from build123d import *

# Parameters (mm, degrees)
CUT_EXTRUDE2_DEPTH      = 10
CUT_EXTRUDE2_DEPTH_BACK = 10
BOSS_EXTRUDE1_START     = -0.2
SKETCH6_R               = 2.5
SKETCH6_R_2             = 1.5
BOSS_EXTRUDE1_DEPTH     = 10


with BuildPart() as part:
    # Sketch1 → Revolve1 (revolve)
    with BuildSketch(Plane(origin=(0, 0, 0), x_dir=(0, 0, -1), z_dir=(1, 0, 0)), mode=Mode.PRIVATE) as revolve1_sk:
        Polygon((6.5, 15.5), (-6.5, 15.5), (-8, 17), (-8, 18.5), (-6.5, 18.5), (-5, 16.5), (5, 16.5), (6.5, 18.5), (8, 18.5), (8, 17), align=None)
    revolve(revolve1_sk.sketch.rotate(Axis((0, 0, 10.557897078), (0, 0, -1)), 90), axis=Axis((0, 0, 10.557897078), (0, 0, -1)))

    # Sketch3 → Revolve2 (revolve)
    with BuildSketch(Plane(origin=(0, 0, 0), x_dir=(0, 0, -1), z_dir=(1, 0, 0)), mode=Mode.PRIVATE) as revolve2_sk:
        with BuildLine():
            Line((-6.25, 4.5), (-6.25, 2.5))
            Line((-6.25, 2.5), (-4.75, 2.5))
            Line((-4.75, 2.5), (-4.75, 0))
            Line((-4.75, 0), (-4, 0))
            Line((-4, 0), (-4, 2.5))
            Line((-4, 2.5), (5.75, 2.5))
            Line((5.75, 2.5), (5.75, 3.25))
            Line((5.75, 3.25), (-5.5, 3.25))
            Line((-5.5, 3.25), (-5.5, 4.5))
            ThreePointArc((-5.5, 4.5), (-7.225700509, 9.988531242), (-6.719669914, 15.719669914))
            Line((-6.719669914, 15.719669914), (-7.25, 16.25))
            ThreePointArc((-7.25, 16.25), (-7.918610158, 10.275543816), (-6.25, 4.5))
        make_face()
    revolve(revolve2_sk.sketch.rotate(Axis((0, 0, 4.75), (0, 0, -1)), 90), axis=Axis((0, 0, 4.75), (0, 0, -1)))

    # Sketch4 → Cut-Extrude2 (cut, two sides: drawn at the far end of the back side and taken through both)
    with BuildSketch(Plane.XY.offset(-CUT_EXTRUDE2_DEPTH_BACK)):
        with BuildLine():
            Line((-1.5, 7.406883651), (-8.150991135, 14.057874786))
            ThreePointArc((-8.150991135, 14.057874786), (0, 16.25), (8.150991135, 14.057874786))
            Line((8.150991135, 14.057874786), (1.5, 7.406883651))
            ThreePointArc((1.5, 7.406883651), (0, 7.557243242), (-1.5, 7.406883651))
        make_face()
        with BuildLine():
            Line((6.58083947, 3.715437698), (10.851038639, 12.096175447))
            ThreePointArc((10.851038639, 12.096175447), (15.45466839, 5.021526159), (15.888628203, -3.40793102))
            Line((15.888628203, -3.40793102), (7.507890453, 0.862268149))
            ThreePointArc((7.507890453, 0.862268149), (7.187365431, 2.335316592), (6.58083947, 3.715437698))
        make_face()
        with BuildLine():
            Line((5.567182467, -5.110616871), (14.857301828, -6.582027226))
            ThreePointArc((14.857301828, -6.582027226), (9.55151035, -13.146526159), (1.668721129, -16.164091988))
            Line((1.668721129, -16.164091988), (3.140131484, -6.873972628))
            ThreePointArc((3.140131484, -6.873972628), (4.442036126, -6.113938214), (5.567182467, -5.110616871))
        make_face()
        with BuildLine():
            Line((-3.140131484, -6.873972628), (-1.668721129, -16.164091988))
            ThreePointArc((-1.668721129, -16.164091988), (-9.55151035, -13.146526159), (-14.857301828, -6.582027226))
            Line((-14.857301828, -6.582027226), (-5.567182467, -5.110616871))
            ThreePointArc((-5.567182467, -5.110616871), (-4.442036126, -6.113938214), (-3.140131484, -6.873972628))
        make_face()
        with BuildLine():
            Line((-7.507890453, 0.862268149), (-15.888628203, -3.40793102))
            ThreePointArc((-15.888628203, -3.40793102), (-15.45466839, 5.021526159), (-10.851038639, 12.096175447))
            Line((-10.851038639, 12.096175447), (-6.58083947, 3.715437698))
            ThreePointArc((-6.58083947, 3.715437698), (-7.187365431, 2.335316592), (-7.507890453, 0.862268149))
        make_face()
    extrude(amount=CUT_EXTRUDE2_DEPTH + CUT_EXTRUDE2_DEPTH_BACK, mode=Mode.SUBTRACT)

    # Sketch5 → Revolve3 (revolve)
    with BuildSketch(Plane(origin=(0, 0, 0), x_dir=(0, 0, -1), z_dir=(1, 0, 0)), mode=Mode.PRIVATE) as revolve3_sk:
        with BuildLine():
            Line((-8.2, 18.5), (-6.5, 18.5))
            Line((-6.5, 18.5), (-5, 16.5))
            Line((-5, 16.5), (5, 16.5))
            Line((5, 16.5), (6.5, 18.5))
            Line((6.5, 18.5), (8.2, 18.5))
            ThreePointArc((8.2, 18.5), (8.553553391, 18.646446609), (8.7, 19))
            Line((8.7, 19), (8.7, 19.5))
            ThreePointArc((8.7, 19.5), (8.553553391, 19.853553391), (8.2, 20))
            Line((8.2, 20), (-8.2, 20))
            ThreePointArc((-8.2, 20), (-8.553553391, 19.853553391), (-8.7, 19.5))
            Line((-8.7, 19.5), (-8.7, 19))
            ThreePointArc((-8.7, 19), (-8.553553391, 18.646446609), (-8.2, 18.5))
        make_face()
    revolve(revolve3_sk.sketch.rotate(Axis((0, 0, 17.280057329), (0, 0, -1)), 90), axis=Axis((0, 0, 17.280057329), (0, 0, -1)))

    # Sketch6 → Boss-Extrude1 (add)
    with BuildSketch(Plane(origin=(0, 0, -5.75), x_dir=(-1, 0, 0), z_dir=(0, 0, -1)).offset(BOSS_EXTRUDE1_START)):
        with Locations(Location((0, 0, 0), (0, 0, 180))):
            Circle(SKETCH6_R)
        Circle(SKETCH6_R_2, mode=Mode.SUBTRACT)
    extrude(amount=-BOSS_EXTRUDE1_DEPTH)


solid = part.part
The listing builds one solid part. Answer for the finished solid, in the listing's coordinates (mm). A direction names the side the tool comes from. Give positions to 0.01 mm unless a question says otherwise; leave off trailing zeros. Use one line per item in the form item = value.
1) Find section A-A on z = 0. Give the number of separate pieces and of enclosed holes in the cut face, and give its area (3 significant figures).
Verdict:
separate_pieces = 2
enclosed_holes = 2
area = 466 mm^2
2) For faces 1 (the cylindrical face through (9.09, 12.555, 0.091)), 2 (the cylindrical face through (-2.5, -0.1, 5.5)), 3 (the cylindrical face through (-7.18, 2.36, 7.09)), determine the directions among +Z, -Z, +X, -X, +Y, -Y from which every point of the face is accessible in a straight line to the end or side of a thin tool.
Verdict:
face_1 = -Z
face_2 = +Z
face_3 = +Z, -Z
3) The mould has two halves that part along X. Classify faces 4 (the flat face through (-4.2, 18.7, -8.7)), 5 (the flat face through (1.747, -15.67, 2.589)), 6 (the cylindrical face through (-19.98, -0.88, 0.11)): released by +X, released by -X, zero draft, split by the parting line, or undercut.
Verdict:
face_4 = zero draft
face_5 = undercut
face_6 = split by the parting line
4) Each of these flat-tipped pins is pushed along its axis until it touches: pin 1 (6 mm diameter, centred on y = 8, z = 0.5, fed in from -X); pin 2 (5.5 mm diameter, centred on x = -0.5, y = -1, fed in from -Z); pin 3 (5 mm diameter, centred on x = 2.5, z = 0.5, fed in from -Y). Where does it stop, or does it pass through?
Verdict:
pin_1 = -19.36
pin_2 = -5.75
pin_3 = -20
5) Consider probe 1 along Y at (x, z) = (0, -2); probe 2 along Y at (x, z) = (0, -8.1); probe 3 along X at (y, z) = (0.5, 2.5). Determine where each line is inside the solid, lowest interval first. Write a range as [from, to].
Verdict:
probe_1 = [-20, -15.5], [-3.25, -1.5], [1.5, 3.25], [16.25, 20]
probe_2 = [-20, -18.5], [18.5, 20]
probe_3 = [-19.99, -16.24], [-3.21, -1.41], [1.41, 3.21], [16.24, 19.99]
